from build123d import *

# Parameters (mm, degrees)
F0_W     = 10
F0_H     = 25.4
F1_DEPTH = 5
F2_R     = 4.99999
F3_R     = 2.25
F4_DEPTH = 0.9
F5_R     = 2.25
F6_DEPTH = 0.9


# Not quite as in the source:
# - a fillet or chamfer is up to 0.001 mm smaller than in the source, because OpenCascade refuses the exact size


with BuildPart() as f1:
    # F0 (on Front) → F1 (new body)
    with BuildSketch(Plane.XZ):
        with Locations((-3.6362301892, -0.5979733542)):
            Rectangle(F0_W, F0_H)
    extrude(amount=F1_DEPTH)

    # F2 (radius 5 in the source; OpenCascade refuses exactly that, so slightly less here)
    f2_edges = [f1.edges().sort_by_distance(p)[0] for p in [
        (1.36377, 0, -0.597973),
        (-8.63623, -5, -0.597973),
    ]]
    fillet(f2_edges, radius=F2_R)

    # F3 (on face) → F4 (cut)
    with BuildSketch(Plane.XY.offset(12.1020266458)):
        with Locations((-3.5037611703, -2.5272680031)):
            Circle(F3_R)
    extrude(amount=-F4_DEPTH, mode=Mode.SUBTRACT)

    # F5 (on face) → F6 (cut)
    with BuildSketch(Plane(origin=(0, 0, -13.2979733542), x_dir=(1, 0, 0), z_dir=(0, 0, -1))):
        with Locations((-3.5220479187, 2.6191056776)):
            Circle(F5_R)
    extrude(amount=-F6_DEPTH, mode=Mode.SUBTRACT)


solid = f1.part
Check sheet for the modelled part. Datum: model origin and axes. Units: mm. A direction names the side the tool comes from. Round coordinates to 2 decimals unless told otherwise and drop trailing zeros. Loops run counter-clockwise (first coordinate to the right, second up) from the corner with the lowest first, then second, coordinate; pieces in that order, holes last.
1. Set-up check for faces 5 (the flat face through (-6, -2, -13.298)), 6 (the cylindrical face through (-5.289, -3.896, 11.658)), 7 (the flat face through (-4, -3, -12.398)): record each of +Z, -Z, +X, -X, +Y, -Y from which the full face is reachable in a straight line by a thin tool's end or side.
2. Scan lines: probe 1 along Z at (x, y) = (-2.5, -3.3); probe 2 along Y at (x, z) = (-2, -3); probe 3 along X at (y, z) = (-4.25, -10.75). Record each from-to range of solid material in increasing order.
3. Mould release check, pull along X, two halves, no side actions. Record for faces 1 (the flat face through (-4, -2, 11.202)), 2 (the cylindrical face through (-0.062, -1.504, -0.42)), 3 (the cylindrical face through (-4.01, -0.423, -12.854)), 4 (the flat face through (-1, -5, 0)): released by +X, released by -X, zero draft, split by the parting line, or undercut.
4. Sectioned sample at D-D on x = -7.5. Record the boundary of the cut face in (y, z).
5. Sectioned sample at A-A on y = -1.7. Record the boundary of the cut face in (x, z), and give its area (3 significant figures).
6. Sectioned sample at B-B on x = -1.5. Record the boundary of the cut face in (y, z), and give its area (3 significant figures).
7. Gauge pin test, flat ends, axial feed: pin 1 Ø2 at (y, z) = (-3.5, -6.5) entering from +X; pin 2 Ø1.3 at (x, y) = (-4, -2.5) entering from -Z; pin 3 Ø1.5 at (x, y) = (-4, -3) entering from +Z. Record the tip position at first contact, or that the pin passes through.
Recorded:
1. face 5: -Z, +X, -X, +Y, -Y
1. face 6: +Z
1. face 7: -Z
2. probe 1: z = -12.4 to 11.2
2. probe 2: y = -5 to -0.28
2. probe 3: x = -6.27 to 1.31
3. face 1: undercut
3. face 2: released by +X
3. face 3: undercut
3. face 4: zero draft
4. outline: (-3.17, -13.3) - (0, -13.3) - (0, 12.1) - (-3.17, 12.1) - close
5. outline: (-8.34, -13.3) - (-5.58, -13.3) - (-5.58, -12.4) - (-1.47, -12.4) - (-1.47, -13.3) - (0.12, -13.3) - (0.12, 12.1) - (-1.41, 12.1) - (-1.41, 11.2) - (-5.6, 11.2) - (-5.6, 12.1) - (-8.34, 12.1) - close
5. area: 207 mm2
6. outline: (-5, -13.3) - (-3.61, -13.3) - (-3.61, -12.4) - (-1.63, -12.4) - (-1.63, -13.3) - (-0.48, -13.3) - (-0.48, 12.1) - (-1.5, 12.1) - (-1.5, 11.2) - (-3.55, 11.2) - (-3.55, 12.1) - (-5, 12.1) - close
6. area: 111 mm2
7. pin 1: stops at x = 1.34
7. pin 2: stops at z = -12.4
7. pin 3: stops at z = 11.2
